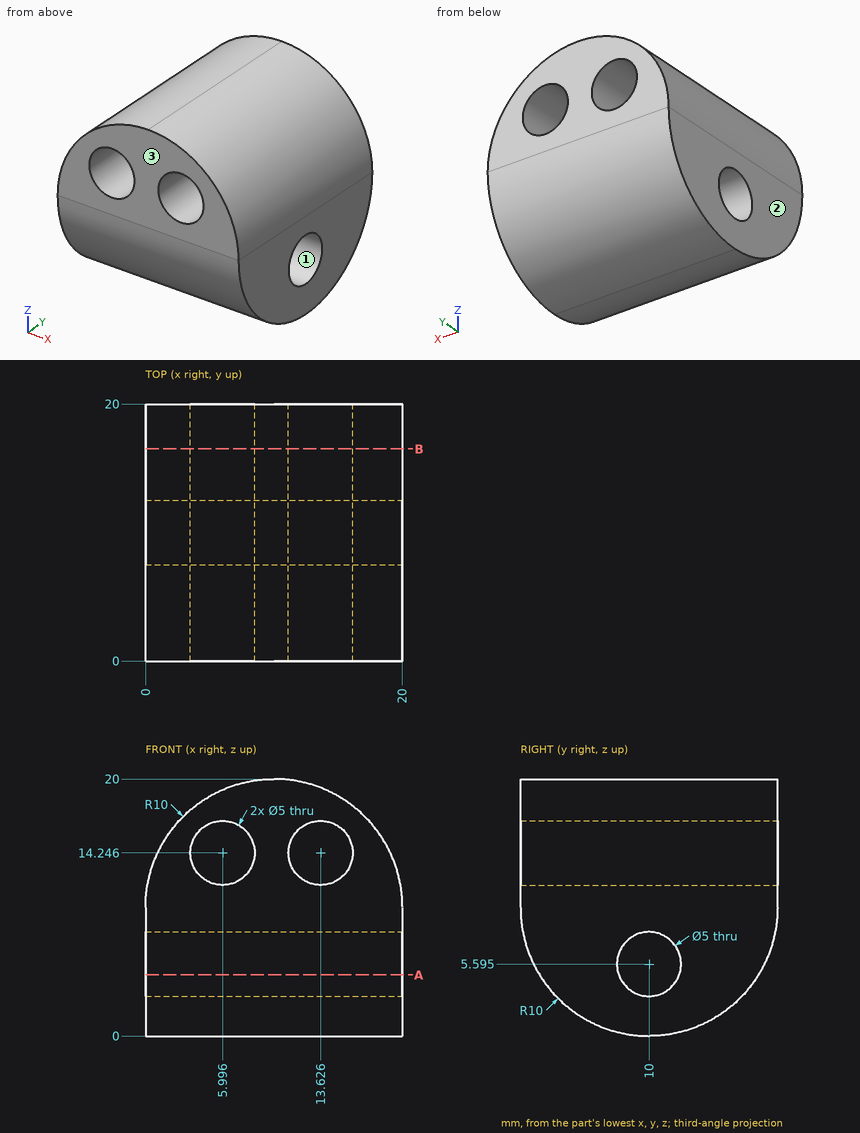
For this review, use the dimensioned drawing (mm, ordinates from the lowest corner) and the shaded views. Give positions to 0.01 mm unless a question says otherwise; leave off trailing zeros. Order: outer loops, then holes, each group sorted by start corner. A loop starts at its lowest first (then second) coordinate and runs counter-clockwise, first axis right, second up. Notation, with made-up numbers: M -5.75,-18 L 40.25,-18 A14 cw 40.25,2 Z; hole C 67.5,-24 d1. An arc over 180 degrees is marked long. Use one line per item in the form item = value. Start each with the question number.
Item 1: We need section A-A on z = 4.75. Give the boundary of the cut face in (x, y), plus the area to 3 significant figures.
Item 2: We need section B-B on y = 16.5. Give the number of separate pieces and of enclosed holes in the cut face, plus the area to 3 significant figures.
Item 3: The part is to be moulded in two halves that separate along Y. For the marked faces 1, 2 and 3, say which applies: pulls with the +Y half, pulls with the -Y half, needs draft (parallel to the pull), parting line crosses it, or undercut.
Item 4: Insertion check: pin 1 Ø4 at (y, z) = (10, 5.6) entering from +X; pin 2 Ø3 at (x, z) = (2, 6) entering from +Y; pin 3 Ø1.5 at (y, z) = (9.5, 11.5) entering from +X; pin 4 Ø2 at (x, y) = (2.5, 14.5) entering from -Z. Each pin has a flat end and moves straight along its axis. Give the tip position at first contact, or say it passes through.
Item 5: To check wall thickness, follow line 1 along Z through (x, y) = (6.5, 10.5) (1 decimal); line 2 along Z through (x, y) = (18.75, 11.75) (1 decimal); line 3 along X through (y, z) = (17.75, 12) (1 decimal). State the ranges of each line that lie inside material, in increasing order. Write a range as from..to.
Completed:
q1.outline = M 0,1.49 L 20,1.49 L 20,7.65 L 0,7.65 Z; M 0,12.35 L 20,12.35 L 20,18.51 L 0,18.51 Z
q1.area = 246 mm²
q2.separate_pieces = 1
q2.enclosed_holes = 2
q2.area = 270 mm²
q3.face_1 = undercut
q3.face_2 = needs draft
q3.face_3 = pulls with the -Y half
q4.pin_1 = through
q4.pin_2 = 19.68
q4.pin_3 = 19.97
q4.pin_4 = 0.63
q5.line_1 = 0..3.1, 8..11.8, 16.7..19.4
q5.line_2 = 0.2..3.8, 7.4..14.8
q5.line_3 = 0.2..4.9, 7.1..12.5, 14.7..19.8
